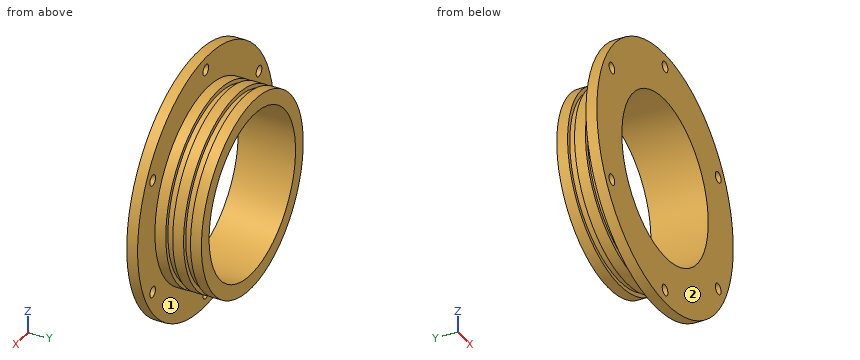
from build123d import *

# Parameters (mm, degrees)
SKETCH1_R           = 60
SKETCH1_R_2         = 38
BOSS_EXTRUDE1_DEPTH = 5
SKETCH2_R           = 44.8
SKETCH2_R_2         = 38
BOSS_EXTRUDE2_DEPTH = 21.4
SKETCH4_R           = 2.5
CUT_EXTRUDE1_DEPTH  = 20


with BuildPart() as part:
    # Sketch1 → Boss-Extrude1 (new body)
    with BuildSketch(Plane(origin=(0, 0, 0), x_dir=(1, 0, 0), z_dir=(0, 1, 0))):
        with Locations(Location((0, 0, 0), (0, 0, 270))):
            Circle(SKETCH1_R)
        with Locations(Location((0, 0, 0), (0, 0, 270))):
            Circle(SKETCH1_R_2, mode=Mode.SUBTRACT)
    extrude(amount=BOSS_EXTRUDE1_DEPTH)

    # Sketch2 → Boss-Extrude2 (add)
    with BuildSketch(Plane(origin=(0, 5, 0), x_dir=(1, 0, 0), z_dir=(0, 1, 0))):
        with Locations(Location((0, 0, 0), (0, 0, 270))):
            Circle(SKETCH2_R)
        with Locations(Location((0, 0, 0), (0, 0, 270))):
            Circle(SKETCH2_R_2, mode=Mode.SUBTRACT)
    extrude(amount=BOSS_EXTRUDE2_DEPTH)

    # Sketch3 → Cut-Revolve1 (revolve, cut)
    with BuildSketch(Plane(origin=(0, 0, 0), x_dir=(0, 0, -1), z_dir=(1, 0, 0)), mode=Mode.PRIVATE) as cut_revolve1_sk:
        Polygon((-45.972863263, 10), (-45.972863263, 18.2), (-45.972863263, 21.4), (-44.8, 21.4), (-42.9, 21.4), (-42.9, 18.2), (-44.8, 18.2), (-44.8, 13.2), (-42.9, 13.2), (-42.9, 10), (-44.8, 10), align=None)
    revolve(cut_revolve1_sk.sketch.rotate(Axis((0, 0, 0), (0, 1, 0)), 180), axis=Axis((0, 0, 0), (0, 1, 0)), mode=Mode.SUBTRACT)

    # Sketch4 → Cut-Extrude1 (cut)
    with BuildSketch(Plane.XZ):
        with Locations(Location((0, 54, 0), (0, 0, 270))):
            Circle(SKETCH4_R)
        with Locations(Location((46.765371804, 27, 0), (0, 0, 270))):
            Circle(SKETCH4_R)
        with Locations(Location((46.765371804, -27, 0), (0, 0, 270))):
            Circle(SKETCH4_R)
        with Locations(Location((0, -54, 0), (0, 0, 270))):
            Circle(SKETCH4_R)
        with Locations(Location((-46.765371804, -27, 0), (0, 0, 270))):
            Circle(SKETCH4_R)
        with Locations(Location((-46.765371804, 27, 0), (0, 0, 270))):
            Circle(SKETCH4_R)
    extrude(amount=-CUT_EXTRUDE1_DEPTH, mode=Mode.SUBTRACT)


solid = part.part
Geometry: final body of the model. Coordinates: model frame, mm. Face numbers are marked on the shaded views. A direction names the side the tool comes from. Give positions to 0.01 mm unless a question says otherwise; leave off trailing zeros. Order: outer loops, then holes, each group sorted by start corner. A loop starts at its lowest first (then second) coordinate and runs counter-clockwise, first axis right, second up. Notation, with made-up numbers: (-14, 56) -> (38, 56) arc R18 cw to (38, 61) -> close; hole circle Ø9 at (0.5, 16.5). An arc over 180 degrees is marked (long way). Write each question's results on one line, items separated by ' | '.
1) Cut plane C-C (y = 16.25). Output: boundary loops of the cut face in (x, z).
Geometry says:
outline: circle Ø89.6 at (0, 0); hole circle Ø76 at (0, 0)
2) Cut plane B-B (x = 7.5). Output: boundary loops of the cut face in (y, z).
Geometry says:
outline: (0, -59.53) -> (5, -59.53) -> (5, -44.17) -> (10, -44.17) -> (10, -42.24) -> (13.2, -42.24) -> (13.2, -44.17) -> (18.2, -44.17) -> (18.2, -42.24) -> (21.4, -42.24) -> (21.4, -44.17) -> (26.4, -44.17) -> (26.4, -37.25) -> (0, -37.25) -> close; (0, 37.25) -> (26.4, 37.25) -> (26.4, 44.17) -> (21.4, 44.17) -> (21.4, 42.24) -> (18.2, 42.24) -> (18.2, 44.17) -> (13.2, 44.17) -> (13.2, 42.24) -> (10, 42.24) -> (10, 44.17) -> (5, 44.17) -> (5, 59.53) -> (0, 59.53) -> close
3) Set-up query: the marked faces 1 and 2. Return all of +Z, -Z, +X, -X, +Y, -Y with unobstructed straight access to the full face (end or side cutting, diameter ignored); none if empty.
Geometry says:
face 1: +Y | face 2: +Z, -Z, +X, -X, -Y
4) Cut plane D-D (z = 27). Give the number of separate pieces and of enclosed holes in the cut face, and give its area (3 significant figures).
Geometry says:
separate pieces: 4 | enclosed holes: 0 | area: 573 mm²
5) Line query: line 1 along Y through (x, z) = (11, -41.5); line 2 along X through (y, z) = (1.15, -27); line 3 along Y through (x, z) = (40.5, -23). Output: solid intervals per line, ascending.
Geometry says:
line 1: y = 0 to 10, 13.2 to 18.2, 21.4 to 26.4 | line 2: x = -53.58 to -49.27, -44.27 to -26.74, 26.74 to 44.27, 49.27 to 53.58 | line 3: y = 0 to 5
6) Cut plane A-A (z = 0). Output: boundary loops of the cut face in (x, y).
Geometry says:
outline: (-60, 0) -> (-38, 0) -> (-38, 26.4) -> (-44.8, 26.4) -> (-44.8, 21.4) -> (-42.9, 21.4) -> (-42.9, 18.2) -> (-44.8, 18.2) -> (-44.8, 13.2) -> (-42.9, 13.2) -> (-42.9, 10) -> (-44.8, 10) -> (-44.8, 5) -> (-60, 5) -> close; (38, 0) -> (60, 0) -> (60, 5) -> (44.8, 5) -> (44.8, 10) -> (42.9, 10) -> (42.9, 13.2) -> (44.8, 13.2) -> (44.8, 18.2) -> (42.9, 18.2) -> (42.9, 21.4) -> (44.8, 21.4) -> (44.8, 26.4) -> (38, 26.4) -> close
7) First-contact query: pin 1 Ø12 at (y, z) = (23, 26.5) entering from -X; pin 2 Ø3 at (x, z) = (0, 54) entering from +Y; pin 3 Ø12 at (x, y) = (-32, 16.5) entering from +Z; pin 4 Ø5 at (y, z) = (21.5, -28.5) entering from +X. Flat tips, straight axial feed; report the tip coordinate or a pass-through.
Geometry says:
pin 1: stops at x = -39.83 | pin 2: passes through | pin 3: stops at z = 36.48 | pin 4: stops at x = 36.48
